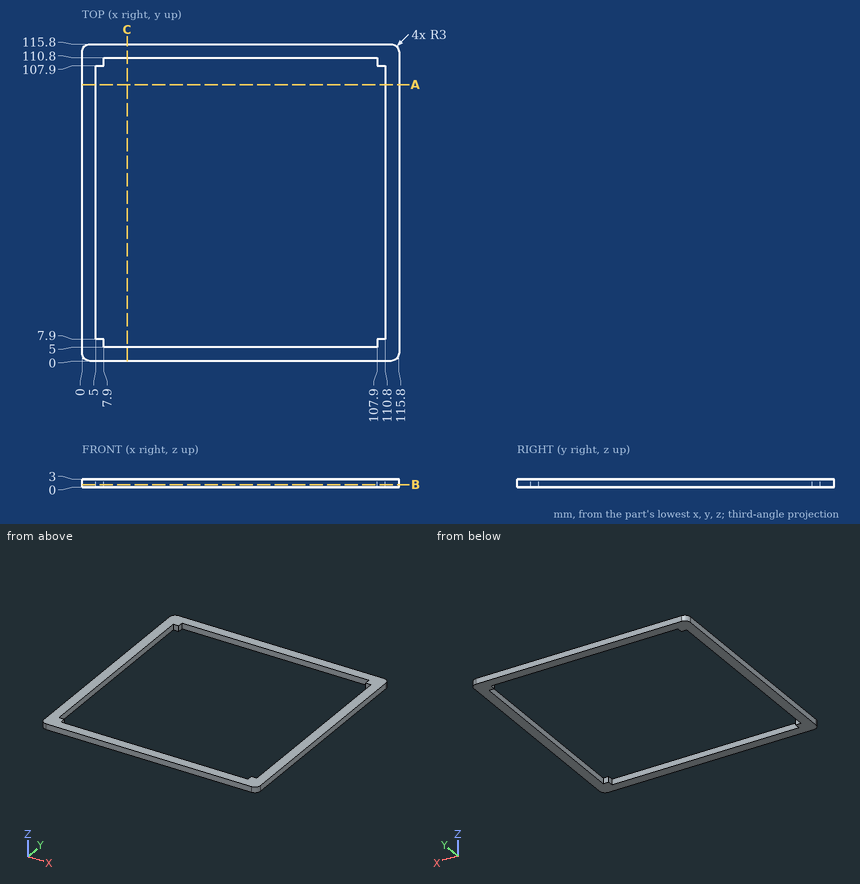
Study the drawing (mm; zero at the part's minimum x, y, z) and answer. Round coordinates to 2 decimals unless told otherwise and drop trailing zeros. Loops run counter-clockwise (first coordinate to the right, second up) from the corner with the lowest first, then second, coordinate; pieces in that order, holes last. Notation, with made-up numbers: (51.25, 55.25) -> (67.25, 55.25) arc R28 cw to (67.25, 85.25) -> close; hole circle Ø9 at (36, -8). An arc over 180 degrees is marked (long way). Use one line per item in the form item = value.
1. Find the intervals of material crossed by probe 1 along X at (y, z) = (11.5, 1.6), in increasing order. Write a range as [from, to].
Answer key:
probe_1 = [0, 5], [110.8, 115.8]
2. The part is cut by section A-A on y = 101. Determine the outline of the cut face in (x, z).
Answer key:
outline = (0, 0) -> (5, 0) -> (5, 3) -> (0, 3) -> close; (110.8, 0) -> (115.8, 0) -> (115.8, 3) -> (110.8, 3) -> close
3. The part is cut by section B-B on z = 0.95. Determine the outline of the cut face in (x, y).
Answer key:
outline = (0, 3) arc R3 ccw to (3, 0) -> (112.8, 0) arc R3 ccw to (115.8, 3) -> (115.8, 112.8) arc R3 ccw to (112.8, 115.8) -> (3, 115.8) arc R3 ccw to (0, 112.8) -> close; hole (5, 7.9) -> (7.9, 7.9) -> (7.9, 5) -> (107.9, 5) -> (107.9, 7.9) -> (110.8, 7.9) -> (110.8, 107.9) -> (107.9, 107.9) -> (107.9, 110.8) -> (7.9, 110.8) -> (7.9, 107.9) -> (5, 107.9) -> close
